```python
from build123d import *

# Parameters (mm, degrees)
F1_DEPTH = 12.7
F2_START = 7.62
F2_DEPTH = 5.08
F3_START = -7.62
F3_DEPTH = 5.08
F4_DEPTH = 7.62


with BuildPart() as f1:
    # F0 (on Right) → F1 (new body, symmetric)
    with BuildSketch(Plane.YZ):
        with BuildLine():
            ThreePointArc((12.7, 0), (14.5598719395, 4.4901280605), (19.05, 6.35))
            Line((19.05, 6.35), (-19.05, 6.35))
            ThreePointArc((-19.05, 6.35), (-14.5598719395, 4.4901280605), (-12.7, 0))
            ThreePointArc((-12.7, 0), (-14.5598719395, -4.4901280605), (-19.05, -6.35))
            Line((-19.05, -6.35), (10.4731516913, -6.35))
            Line((10.4731516913, -6.35), (12.7, 0))
        make_face()
    extrude(amount=F1_DEPTH, both=True)

    # F0 (on Right) → F2 (join)
    with BuildSketch(Plane.YZ.offset(F2_START)):
        with BuildLine():
            ThreePointArc((25.4, 0), (23.5401280605, 4.4901280605), (19.05, 6.35))
            Line((19.05, 6.35), (19.05, -6.35))
            ThreePointArc((19.05, -6.35), (23.5401280605, -4.4901280605), (25.4, 0))
        make_face()
        with BuildLine():
            Line((19.05, -6.35), (19.05, 6.35))
            ThreePointArc((19.05, 6.35), (14.5598719395, 4.4901280605), (12.7, 0))
            ThreePointArc((12.7, 0), (14.5598719395, -4.4901280605), (19.05, -6.35))
        make_face()
    extrude(amount=F2_DEPTH)

    # F0 (on Right) → F3 (join)
    with BuildSketch(Plane.YZ.offset(F3_START)):
        with BuildLine():
            ThreePointArc((25.4, 0), (23.5401280605, 4.4901280605), (19.05, 6.35))
            Line((19.05, 6.35), (19.05, -6.35))
            ThreePointArc((19.05, -6.35), (23.5401280605, -4.4901280605), (25.4, 0))
        make_face()
        with BuildLine():
            Line((19.05, -6.35), (19.05, 6.35))
            ThreePointArc((19.05, 6.35), (14.5598719395, 4.4901280605), (12.7, 0))
            ThreePointArc((12.7, 0), (14.5598719395, -4.4901280605), (19.05, -6.35))
        make_face()
    extrude(amount=-F3_DEPTH)

    # F0 (on Right) → F4 (join, symmetric)
    with BuildSketch(Plane.YZ):
        with BuildLine():
            ThreePointArc((-12.7, 0), (-14.5598719395, 4.4901280605), (-19.05, 6.35))
            Line((-19.05, 6.35), (-19.05, -6.35))
            ThreePointArc((-19.05, -6.35), (-14.5598719395, -4.4901280605), (-12.7, 0))
        make_face()
        with BuildLine():
            Line((-19.05, -6.35), (-19.05, 6.35))
            ThreePointArc((-19.05, 6.35), (-25.4, 0), (-19.05, -6.35))
        make_face()
    extrude(amount=F4_DEPTH, both=True)


solid = f1.part
```
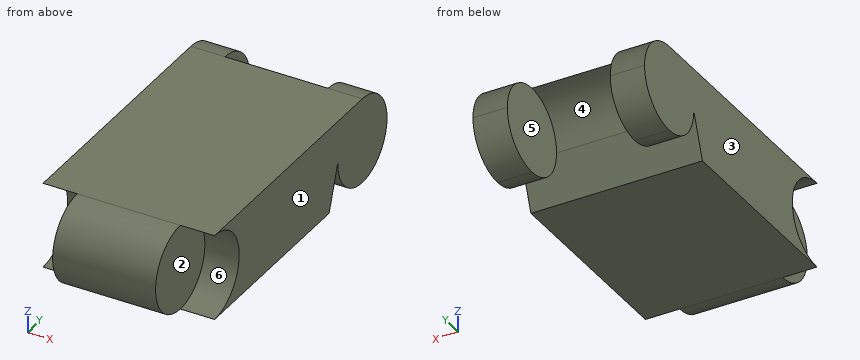
Design review of the part built by this model. Coordinates are the model's own, in mm. Face numbers are marked on the shaded views. A direction names the side the tool comes from. Coordinates: 2 decimals unless noted, no trailing zeros. Write each loop counter-clockwise with the first axis right and the second up, starting at its lowest first coordinate (ties: lowest second). Pieces come first, ordered by that corner, then holes. Notation, with made-up numbers: M 41.5,-32.5 L 70.5,-32.5 A4 cw 70.5,-25.5 Z; hole C -6.75,-31 d7. An arc over 180 degrees is marked long. Answer as a JSON object with one key per item and string values.
Item 1: Add section C-C, the plane y = 17.5. Give the boundary of the cut face in (x, z), and give its area (3 significant figures).
Outcome:
{"outline": "M -12.7,-6.16 L -7.62,-6.16 L -7.62,6.16 L 7.62,6.16 L 7.62,-6.16 L 12.7,-6.16 L 12.7,6.35 L -12.7,6.35 Z", "area": "130 mm²"}
Item 2: Insertion check: pin 1 Ø4 at (y, z) = (-17.5, 1.5) entering from -X; pin 2 Ø2 at (x, z) = (8.5, 0.5) entering from +Y; pin 3 Ø1 at (x, z) = (7.5, -2) entering from +Y; pin 4 Ø4 at (y, z) = (-22, 1) entering from +X. Each pin has a flat end and moves straight along its axis. Give the tip position at first contact, or say it passes through.
Outcome:
{"pin 1": "x = -7.62", "pin 2": "y = 25.4", "pin 3": "y = 25.22", "pin 4": "x = 7.62"}
Item 3: Wall thickness on probe 1 along X at (y, z) = (20.5, 4.5); probe 2 along X at (y, z) = (-18, -0.5); probe 3 along Y at (x, z) = (10.5, -2.75): over which ranges is each line inside the solid? List them lowest first.
Outcome:
{"probe 1": "-12.7 to -7.62, 7.62 to 12.7", "probe 2": "-7.62 to 7.62", "probe 3": "-13.33 to 11.74, 13.33 to 24.77"}
Item 4: Add section D-D, the plane z = 0.5. Give the boundary of the cut face in (x, y), and give its area (3 significant figures).
Outcome:
{"outline": "M -12.7,-12.72 L -7.62,-12.72 L -7.62,-25.38 L 7.62,-25.38 L 7.62,-12.72 L 12.7,-12.72 L 12.7,25.38 L 7.62,25.38 L 7.62,12.72 L -7.62,12.72 L -7.62,25.38 L -12.7,25.38 Z", "area": "968 mm²"}
Item 5: Add section B-B, the plane x = -2.25. Give the boundary of the cut face in (y, z), and give its area (3 significant figures).
Outcome:
{"outline": "M -19.05,-6.35 L 10.47,-6.35 L 12.7,0 A6.35 cw 19.05,6.35 L -19.05,6.35 A6.35 ccw Z", "area": "468 mm²"}
Item 6: Machinability: for the marked faces 1 and 2, which of the approach directions +Z, -Z, +X, -X, +Y, -Y give a long, thin tool a straight path to every point of the face, cutting with its end or side? Answer none if there is none.
Outcome:
{"face 1": "+Z, -Z, +X, +Y, -Y", "face 2": "+X, -Y"}
Item 7: Add section A-A, the plane z = -3.5. Give the boundary of the cut face in (x, y).
Outcome:
{"outline": "M -12.7,-13.75 L -7.62,-13.75 L -7.62,-24.35 L 7.62,-24.35 L 7.62,-13.75 L 12.7,-13.75 L 12.7,11.47 L -12.7,11.47 Z; M -12.7,13.75 L -7.62,13.75 L -7.62,24.35 L -12.7,24.35 Z; M 7.62,13.75 L 12.7,13.75 L 12.7,24.35 L 7.62,24.35 Z"}
Item 8: Draft analysis for pull direction X (two halves, no side actions). For the marked faces 3, 4, 5 and 6, state which applies: pulls with the +X half, pulls with the -X half, needs draft (parallel to the pull), parting line crosses it, or undercut.
Outcome:
{"face 3": "pulls with the -X half", "face 4": "undercut", "face 5": "undercut", "face 6": "needs draft"}
